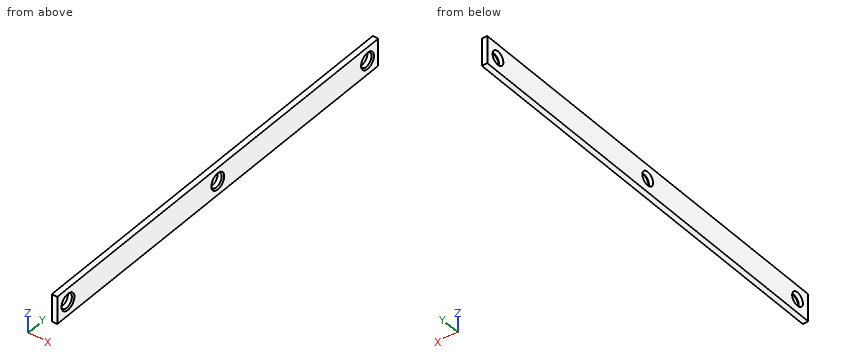
```python
from build123d import *

# Parameters (mm, degrees)
SKETCH_1_W          = 4
SKETCH_1_H          = 20
EXTRUDE_1_DEPTH     = 300
SKETCH_2_R          = 5
CUT_EXTRUDE_1_DEPTH = 5
CHAMFER_1_SIZE      = 1


with BuildPart() as part:
    # Эскиз1 → Бобышка-Вытянуть1 (new body)
    with BuildSketch(Plane(origin=(0, 0, 0), x_dir=(1, 0, 0), z_dir=(0, 1, 0))):
        Rectangle(SKETCH_1_W, SKETCH_1_H)
    extrude(amount=EXTRUDE_1_DEPTH)

    # Эскиз2 → Вырез-Вытянуть1 (cut, through all)
    with BuildSketch(Plane(origin=(2, 0, 0), x_dir=(0, 0, -1), z_dir=(1, 0, 0))):
        with Locations((0, 290)):
            Circle(SKETCH_2_R)
        with Locations((0, 150)):
            Circle(SKETCH_2_R)
        with Locations((0, 10)):
            Circle(SKETCH_2_R)
    extrude(amount=-CUT_EXTRUDE_1_DEPTH, mode=Mode.SUBTRACT)

    # Фаска1
    chamfer_1_edges = [part.edges().sort_by_distance(p)[0] for p in [
        (2, 290, 5),
        (2, 150, 5),
        (2, 10, 5),
    ]]
    chamfer(chamfer_1_edges, length=CHAMFER_1_SIZE)


solid = part.part
```
Part model, mm, in its own coordinate system. Coordinates: 2 decimals unless noted, no trailing zeros. Write each loop counter-clockwise with the first axis right and the second up, starting at its lowest first coordinate (ties: lowest second). Pieces come first, ordered by that corner, then holes.
Item 1: Probe line 1 (Y direction, x = -1.25, z = 0); line 2 (Y direction, x = -1.05, z = -4); line 3 (Z direction, x = 0.45, y = 290). List the from-to ranges inside material, lowest first.
Item 2: Slice it at A-A (z = 0). Write the cut outline in (x, y), and give its area (3 significant figures).
Item 3: Slice it at B-B (y = 290). Write the cut outline in (x, z).
Item 4: Pin check, flat tip, straight feed: pin 1 (6 mm diameter, centred on y = 150, z = 0, fed in from +X). Stop position of the tip, or through.
Item 5: Slice it at C-C (x = -0.2). Write the cut outline in (y, z).
Results found:
1. line 1: y = 0 to 5, 15 to 145, 155 to 285, 295 to 300
1. line 2: y = 0 to 7, 13 to 147, 153 to 287, 293 to 300
1. line 3: z = -10 to -5, 5 to 10
2. outline: (-2, 0) - (2, 0) - (2, 4) - (1, 5) - (-2, 5) - close; (-2, 15) - (1, 15) - (2, 16) - (2, 144) - (1, 145) - (-2, 145) - close; (-2, 155) - (1, 155) - (2, 156) - (2, 284) - (1, 285) - (-2, 285) - close; (-2, 295) - (1, 295) - (2, 296) - (2, 300) - (-2, 300) - close
2. area: 1,080 mm2
3. outline: (-2, -10) - (2, -10) - (2, -6) - (1, -5) - (-2, -5) - close; (-2, 5) - (1, 5) - (2, 6) - (2, 10) - (-2, 10) - close
4. pin 1: passes through
5. outline: (0, -10) - (300, -10) - (300, 10) - (0, 10) - close; hole circle Ø10 at (10, 0); hole circle Ø10 at (150, 0); hole circle Ø10 at (290, 0)
